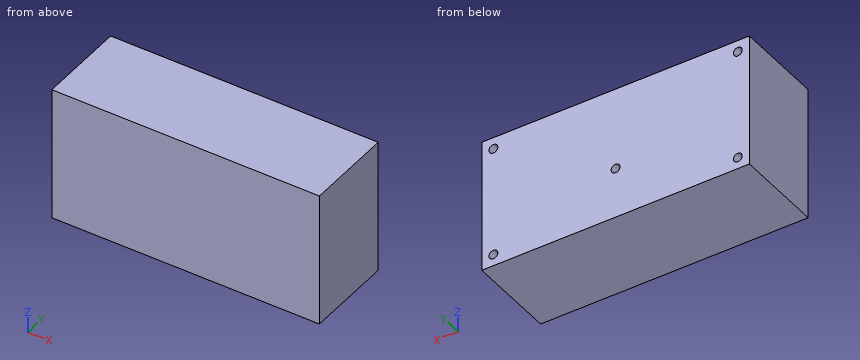
Autodesk Inventor part; units mm, degrees
ref_plane "YZ Plane" through (0, 0, 0) normal (1, 0, 0) x (0, 1, 0)
ref_plane "XZ Plane" through (0, 0, 0) normal (0, 1, 0) x (-1, 0, 0)
ref_plane "XY Plane" through (0, 0, 0) normal (0, 0, 1) x (1, 0, 0)
sketch "Sketch1" plane through (0, 0, 0) normal (0, 1, 0) x (-1, 0, 0)
  line L0 (0, -37.5) -> (-75, -37.5)
  line L1 (-75, -37.5) -> (-75, 0)
  line L2 (-75, 0) -> (0, 0)
  line L3 (0, 0) -> (0, -37.5)
  line L4 (-3.25, -34.25) -> (-71.75, -34.25) construction
  line L5 (-71.75, -34.25) -> (-71.75, -3.25) construction
  line L6 (-71.75, -3.25) -> (-3.25, -3.25) construction
  line L7 (-3.25, -3.25) -> (-3.25, -34.25) construction
  circle A0 centre (-3.25, -34.25) radius 1.25
  circle A1 centre (-37.5, -23.25) radius 1.25
  circle A2 centre (-3.25, -3.25) radius 1.25
  circle A3 centre (-71.75, -3.25) radius 1.25
  circle A4 centre (-71.75, -34.25) radius 1.25
  point P0 (-37.5, -34.25)
  point P1 (-37.5, -37.5)
  point P2 (-3.25, -18.75)
  point P3 (0, -18.75)
  dimension "d0" = 37.5
  dimension "d1" = 75
  dimension "d2" = 31
  dimension "d3" = 68.5
  dimension "d4" = 2.5
  dimension "d6" = 2.5
  dimension "d7" = 2.5
  dimension "d8" = 2.5
  dimension "d9" = 2.5
  dimension "d10" = 34.25
  dimension "d11" = 11
extrude "Extrusion1" add sketch "Sketch1" against normal blind 25 contours L0 L1 L2 L3 | A0 | A1 | A2 | A3 | A4
extrude "Extrusion2" cut sketch "Sketch1" against normal blind 8 contours A0 | A1 | A2 | A3 | A4
properties part number "heatsink-CNC"
CAD build for the part. Positions are in the model's coordinates, mm. Give positions to 0.01 mm unless a question says otherwise; leave off trailing zeros. Write each loop counter-clockwise with the first axis right and the second up, starting at its lowest first coordinate (ties: lowest second). Pieces come first, ordered by that corner, then holes. Notation, with made-up numbers: (66, -33) -> (113, -33) arc R27 cw to (113, -8) -> close; hole circle Ø2 at (9, 77). An arc over 180 degrees is marked (long way). Write each question's results on one line, items separated by ' | '.
1. Drop flat-ended pins along their axis: P1, Ø3, axis at x = 72, z = -3, coming from the +Y side; P2, Ø2, axis at x = 71.75, z = -3.25, coming from the +Y side. Give the stop position or say it passes through.
Geometry check:
P1: y = 0 | P2: y = -8
2. Cut at A-A, the plane x = 37.5. Write the cut outline in (y, z), then the cut area to 4 significant figures.
Geometry check:
outline: (-25, -37.5) -> (0, -37.5) -> (0, -24.5) -> (-8, -24.5) -> (-8, -22) -> (0, -22) -> (0, 0) -> (-25, 0) -> close | area: 917.5 mm²
3. Wall check: probe 1 along Z at (x, y) = (71.75, -3.75); probe 2 along X at (y, z) = (-6, -2.5). Give the ranges that are in metal, low to high. Write a range as [from, to].
Geometry check:
probe 1: [-37.5, -35.5], [-33, -4.5], [-2, 0] | probe 2: [0, 2.25], [4.25, 70.75], [72.75, 75]
4. Cut at C-C, the plane x = 3.25. Write the cut outline in (y, z).
Geometry check:
outline: (-25, -37.5) -> (0, -37.5) -> (0, -35.5) -> (-8, -35.5) -> (-8, -33) -> (0, -33) -> (0, -4.5) -> (-8, -4.5) -> (-8, -2) -> (0, -2) -> (0, 0) -> (-25, 0) -> close
5. Cut at B-B, the plane z = -3.25. Write the cut outline in (x, y), then the cut area to 4 significant figures.
Geometry check:
outline: (0, -25) -> (75, -25) -> (75, 0) -> (73, 0) -> (73, -8) -> (70.5, -8) -> (70.5, 0) -> (4.5, 0) -> (4.5, -8) -> (2, -8) -> (2, 0) -> (0, 0) -> close | area: 1,835 mm²
